from build123d import *

# Parameters (mm, degrees)
SKETCH1_W           = 149
SKETCH1_H           = 96
BOSS_EXTRUDE1_DEPTH = 20.15
SKETCH2_W           = 20
SKETCH2_H           = 25
BOSS_EXTRUDE2_DEPTH = 3
FILLET1_R           = 3
FILLET2_R           = 3
FILLET3_R           = 3


with BuildPart() as part:
    # Sketch1 → Boss-Extrude1 (new body, symmetric)
    with BuildSketch(Plane.XY):
        Rectangle(SKETCH1_W, SKETCH1_H)
    extrude(amount=BOSS_EXTRUDE1_DEPTH, both=True)

    # Sketch2 → Boss-Extrude2 (add, symmetric)
    with BuildSketch(Plane(origin=(0, 48, 0), x_dir=(1, 0, 0), z_dir=(0, 1, 0))):
        with Locations((-57.5, 0)):
            Rectangle(SKETCH2_W, SKETCH2_H)
        with Locations((57.5, 0)):
            Rectangle(SKETCH2_W, SKETCH2_H)
    extrude(amount=BOSS_EXTRUDE2_DEPTH, both=True)

    # Fillet1
    fillet1_edges = [part.edges().sort_by_distance(p)[0] for p in [
        (74.5, 0, 20.15),
        (-74.5, 0, 20.15),
        (74.5, 0, -20.15),
        (-74.5, 0, -20.15),
    ]]
    fillet(fillet1_edges, radius=FILLET1_R)

    # Fillet2
    fillet2_edges = [part.edges().sort_by_distance(p)[0] for p in [
        (0, -48, 20.15),
        (0, -48, -20.15),
        (74.5, -48, 0),
        (-74.5, -48, 0),
        (73.621320344, -48, 19.271320344),
        (73.621320344, -48, -19.271320344),
        (-73.621320344, -48, -19.271320344),
        (-73.621320344, -48, 19.271320344),
    ]]
    fillet(fillet2_edges, radius=FILLET2_R)

    # Fillet3
    fillet3_edges = [part.edges().sort_by_distance(p)[0] for p in [
        (-67.5, 49.5, -12.5),
        (-67.5, 49.5, 12.5),
        (-47.5, 49.5, 12.5),
        (-47.5, 49.5, -12.5),
        (67.5, 49.5, 12.5),
        (67.5, 49.5, -12.5),
        (47.5, 49.5, -12.5),
        (47.5, 49.5, 12.5),
    ]]
    fillet(fillet3_edges, radius=FILLET3_R)


solid = part.part
The model under review builds one solid part; all positions refer to its coordinate system, in mm. A direction names the side the tool comes from. Round coordinates to 2 decimals unless told otherwise and drop trailing zeros. Loops run counter-clockwise (first coordinate to the right, second up) from the corner with the lowest first, then second, coordinate; pieces in that order, holes last. Notation, with made-up numbers: M 72.25,48.25 L 130.25,48.25 A17 cw 130.25,69.25 Z; hole C 86,61.25 d11. An arc over 180 degrees is marked long. Answer as a JSON object with one key per item and string values.
Item 1: The part is to be moulded in two halves that separate along X. For faces 1 (the face through (-48.4, 49.48, -11.64)), 2 (the face through (-58, 49, -12.5)), 3 (the face through (-74.5, 1, 0)), say which applies: +X half, -X half, draft (parallel to the pull), parting line (faces both ways), or undercut.
Check sheet entries:
{"face 1": "undercut", "face 2": "draft", "face 3": "-X half"}
Item 2: For line 1 along Y through (x, z) = (5, 1); line 2 along X through (y, z) = (-38.5, -17.5); line 3 along X through (y, z) = (-13, -18), list the stretches that pass through material, from the lowest coordinate up.
Check sheet entries:
{"line 1": "-48 to 48", "line 2": "-74.48 to 74.48", "line 3": "-74.38 to 74.38"}
Item 3: Tool access review of faces 4 (the face through (-67.5, 49, 0)), 5 (the face through (-58, 49, 12.5)), 6 (the face through (-47.5, 49, 0)), 7 (the face through (48.4, 49.48, -11.64)): name each direction out of +Z, -Z, +X, -X, +Y, -Y from which nothing blocks a thin tool from reaching the whole face with its end or side.
Check sheet entries:
{"face 4": "+Z, -Z, -X, +Y", "face 5": "+Z, +X, -X, +Y", "face 6": "+Z, -Z, +Y", "face 7": "-Z, +Y"}
Item 4: We need section A-A, the plane z = 2.5. State the section outline as (x, y) points, and give its area (3 significant figures).
Check sheet entries:
{"outline": "M -74.5,-45 A3 ccw -71.5,-48 L 71.5,-48 A3 ccw 74.5,-45 L 74.5,48 L 67.5,48 L 67.5,51 L 47.5,51 L 47.5,48 L -47.5,48 L -47.5,51 L -67.5,51 L -67.5,48 L -74.5,48 Z", "area": "14,400 mm2"}
Item 5: Clearance check with flat-ended pins moving along their axes: P1, Ø0.9, axis at x = -58, y = 49.5, coming from the -Z side; P2, Ø2.5, axis at y = 50, z = 0, coming from the -X side; P3, Ø0.9, axis at x = 60, y = 50, coming from the +Z side. State where each tip first meets the part, or that it passes through.
Check sheet entries:
{"P1": "z = -12.5", "P2": "x = -67.5", "P3": "z = 12.5"}
Item 6: We need section B-B, the plane x = -28.5. State the section outline as (y, z) points.
Check sheet entries:
{"outline": "M -48,-17.15 A3 ccw -45,-20.15 L 48,-20.15 L 48,20.15 L -45,20.15 A3 ccw -48,17.15 Z"}
